```python
from build123d import *

# Parameters (mm, degrees)
SKETCH_1_W                   = 172
SKETCH_1_H                   = 142
EXTRUDE_1_DEPTH              = 6
HOLE_WIZARD_M8_1_D           = 6.8
HOLE_WIZARD_M8_1_DEPTH       = 6
HOLE_WIZARD_M8_1_CSINK_D     = 8.05
HOLE_WIZARD_M8_1_CSINK_ANGLE = 90
HOLE_WIZARD_M8_1_TIP         = 2.042926105
SKETCH_11_R                  = 15
EXTRUDE_3_DEPTH              = 4
SKETCH_12_R                  = 8
CUT_EXTRUDE_1_DEPTH          = 224.266656713


with BuildPart() as part:
    # 草图1 → 凸台-拉伸1 (new body)
    with BuildSketch(Plane.XY):
        with Locations((86, -71)):
            Rectangle(SKETCH_1_W, SKETCH_1_H)
    extrude(amount=EXTRUDE_1_DEPTH)

    # M8 螺纹孔1
    with Locations(Plane.XY.offset(6)):
        with Locations((14, -46), (14, -96), (86, -14), (86, -128), (158, -96), (158, -46)):
            CounterSinkHole(HOLE_WIZARD_M8_1_D / 2, HOLE_WIZARD_M8_1_CSINK_D / 2, depth=HOLE_WIZARD_M8_1_DEPTH, counter_sink_angle=HOLE_WIZARD_M8_1_CSINK_ANGLE)
            with Locations((0, 0, -(HOLE_WIZARD_M8_1_DEPTH + HOLE_WIZARD_M8_1_TIP / 2))):  # 118° drill point
                Cone(0, HOLE_WIZARD_M8_1_D / 2, HOLE_WIZARD_M8_1_TIP, mode=Mode.SUBTRACT)

    # 草图11 → 凸台-拉伸3 (add)
    with BuildSketch(Plane.XY.offset(6)):
        with Locations((86, -71)):
            Circle(SKETCH_11_R)
    extrude(amount=EXTRUDE_3_DEPTH)

    # 草图12 → 切除-拉伸1 (cut, through all)
    with BuildSketch(Plane.XY.offset(10)):
        with Locations((86, -71)):
            Circle(SKETCH_12_R)
    extrude(amount=-CUT_EXTRUDE_1_DEPTH, mode=Mode.SUBTRACT)


solid = part.part
```
The model under review builds one solid part; all positions refer to its coordinate system, in mm. A direction names the side the tool comes from. Round coordinates to 2 decimals unless told otherwise and drop trailing zeros. Write each loop counter-clockwise with the first axis right and the second up, starting at its lowest first coordinate (ties: lowest second). Pieces come first, ordered by that corner, then holes.
(1) Wall thickness on L1, parallel to Y at x = 14, z = 3.45; L2, parallel to X at y = -46, z = 0.75; L3, parallel to Y at x = 86, z = 4.25: over which ranges is each line inside the solid? List them lowest first.
(2) Mouldability with a two-part tool opening along X and no side actions: class faces 3 (the flat face through (85, 0, 3)), 4 (the cylindrical face through (14.44, -42.63, 2.65)), 5 (the flat face through (172, -72, 3)), 6 (the flat face through (0, -72, 3)) as +X half, -X half, draft (parallel to the pull), parting line (faces both ways), or undercut.
(3) We need section B-B on x = 158. Give the boundary of the cut face in (y, z) (3 decimals), and give its area (3 significant figures).
(4) We need section D-D on y = -46. Give the boundary of the cut face in (x, z) (3 decimals), and give its area (3 significant figures).
(5) We need section C-C on z = 1.5. Give the boundary of the cut face in (x, y), and give its area (3 significant figures).
(6) Insertion check: pin 1 (9.5 mm diameter, centred on x = 86, y = -71, fed in from +Z); pin 2 (1.5 mm diameter, centred on y = -86, z = 4.5, fed in from -X); pin 3 (2 mm diameter, centred on x = 60.5, y = -86, fed in from +Z). Each pin has a flat end and moves straight along its axis. Give the tip position at first contact, or say it passes through.
(7) Machinability: for faces 1 (the flat face through (85, -142, 3)), 2 (the cylindrical face through (92.92, -84.31, 7.97)), which of the approach directions +Z, -Z, +X, -X, +Y, -Y give a long, thin tool a straight path to every point of the face, cutting with its end or side? Answer none if there is none.
(8) We need section A-A on y = -71. Give the boundary of the cut face in (x, z).
Findings below:
1. L1: y = -142 to -99.4, -92.6 to -49.4, -42.6 to 0
1. L2: x = 0 to 10.6, 17.4 to 154.6, 161.4 to 172
1. L3: y = -142 to -131.4, -124.6 to -79, -63 to -17.4, -10.6 to 0
2. face 3: draft
2. face 4: undercut
2. face 5: +X half
2. face 6: -X half
3. outline: (-142, 0) - (-99.4, 0) - (-99.4, 5.375) - (-100.025, 6) - (-142, 6) - close; (-92.6, 0) - (-49.4, 0) - (-49.4, 5.375) - (-50.025, 6) - (-91.975, 6) - (-92.6, 5.375) - close; (-42.6, 0) - (0, 0) - (0, 6) - (-41.975, 6) - (-42.6, 5.375) - close
3. area: 770 mm2
4. outline: (0, 0) - (10.6, 0) - (10.6, 5.375) - (9.975, 6) - (0, 6) - close; (17.4, 0) - (154.6, 0) - (154.6, 5.375) - (153.975, 6) - (18.025, 6) - (17.4, 5.375) - close; (161.4, 0) - (172, 0) - (172, 6) - (162.025, 6) - (161.4, 5.375) - close
4. area: 950 mm2
5. outline: (0, -142) - (172, -142) - (172, 0) - (0, 0) - close; hole circle Ø6.8 at (14, -96); hole circle Ø6.8 at (14, -46); hole circle Ø16 at (86, -71); hole circle Ø6.8 at (86, -128); hole circle Ø6.8 at (86, -14); hole circle Ø6.8 at (158, -96); hole circle Ø6.8 at (158, -46)
5. area: 24,000 mm2
6. pin 1: passes through
6. pin 2: stops at x = 0
6. pin 3: stops at z = 6
7. face 1: +Z, -Z, +X, -X, -Y
7. face 2: +Z
8. outline: (0, 0) - (78, 0) - (78, 10) - (71, 10) - (71, 6) - (0, 6) - close; (94, 0) - (172, 0) - (172, 6) - (101, 6) - (101, 10) - (94, 10) - close
